Could you check a few things on this model? Use its own coordinates, in mm. Coordinates: 2 decimals unless noted, no trailing zeros. Loops run counter-clockwise (first coordinate to the right, second up) from the corner with the lowest first, then second, coordinate; pieces in that order, holes last. Notation, with made-up numbers: (-23, -13.5) - (-5, -13.5) arc R5 ccw to (-5, -7.5) - close; hole circle Ø2 at (58.5, 44). An arc over 180 degrees is marked (long way). Put each result on its own line as item: value. Start each with the question number.
```python
from build123d import *

# Parameters (mm, degrees)
SKETCH_1_R      = 5
SKETCH_1_R_2    = 2
EXTRUDE_1_DEPTH = 5


with BuildPart() as part:
    # 草图1 → 凸台-拉伸1 (new body)
    with BuildSketch(Plane(origin=(0, 0, 0), x_dir=(0, 0, -1), z_dir=(1, 0, 0))):
        with BuildLine():
            Line((-7, 33), (-7, 0))
            Line((-7, 0), (7, 0))
            Line((7, 0), (7, 33))
            ThreePointArc((7, 33), (0, 40), (-7, 33))
        make_face()
        with Locations((0, 33)):
            Circle(SKETCH_1_R, mode=Mode.SUBTRACT)
        with Locations((0, 13)):
            Circle(SKETCH_1_R_2, mode=Mode.SUBTRACT)
        with Locations((0, 7)):
            Circle(SKETCH_1_R_2, mode=Mode.SUBTRACT)
    extrude(amount=EXTRUDE_1_DEPTH)


solid = part.part
```
(1) I need wall thicknesses on L1, parallel to Y at x = 3.6, z = 0; L2, parallel to Y at x = 3.8, z = -1.5; L3, parallel to Z at x = 0.9, y = 31. Which ranges of each line are inside material? Lowest first, please. Write a range as [from, to].
(2) For pin 1 Ø2 at (x, z) = (2, -4.5) entering from +Y; pin 2 Ø1.5 at (x, z) = (1, 4) entering from +Y; pin 3 Ø1.5 at (x, z) = (2, -1) entering from -Y, each with a flat end and sliding along its axis, tell me the tip position at first contact or that it passes through.
(3) I want a section at A-A on y = 7. List the corners of the cut face in (x, z) for me.
(4) I want a section at B-B on z = 0. List the corners of the cut face in (x, y) for me, and give its area (3 significant figures).
(5) I want a section at C-C on x = 3.25. List the corners of the cut face in (y, z) for me, and give its area (3 significant figures).
(6) I want a section at D-D on z = -1.5. List the corners of the cut face in (x, y) for me, and give its area (3 significant figures).
(7) If we mould it in two halves opening along Y, with no side actions, what happens to faces 1 (the cylindrical face through (2, 40, 0)), 2 (the cylindrical face through (2, 37, -3)), 3 (the cylindrical face through (2, 15, 0)), 4 (the flat face through (2, 0, 0))? For each: pulls with the +Y half, pulls with the -Y half, needs draft (parallel to the pull), parting line crosses it, or undercut.
Answer sheet:
1. L1: y = [0, 5], [9, 11], [15, 28], [38, 40]
1. L2: y = [0, 5.68], [8.32, 11.68], [14.32, 28.23], [37.77, 39.84]
1. L3: z = [-7, -4.58], [4.58, 7]
2. pin 1: stops at y = 39.06
2. pin 2: stops at y = 39.2
2. pin 3: stops at y = 0
3. outline: (0, -7) - (5, -7) - (5, -2) - (0, -2) - close; (0, 2) - (5, 2) - (5, 7) - (0, 7) - close
4. outline: (0, 0) - (5, 0) - (5, 5) - (0, 5) - close; (0, 9) - (5, 9) - (5, 11) - (0, 11) - close; (0, 15) - (5, 15) - (5, 28) - (0, 28) - close; (0, 38) - (5, 38) - (5, 40) - (0, 40) - close
4. area: 110 mm^2
5. outline: (0, -7) - (33, -7) arc R7 ccw to (33, 7) - (0, 7) - close; hole circle Ø4 at (7, 0); hole circle Ø4 at (13, 0); hole circle Ø10 at (33, 0)
5. area: 435 mm^2
6. outline: (0, 0) - (5, 0) - (5, 5.68) - (0, 5.68) - close; (0, 8.32) - (5, 8.32) - (5, 11.68) - (0, 11.68) - close; (0, 14.32) - (5, 14.32) - (5, 28.23) - (0, 28.23) - close; (0, 37.77) - (5, 37.77) - (5, 39.84) - (0, 39.84) - close
6. area: 125 mm^2
7. face 1: pulls with the +Y half
7. face 2: undercut
7. face 3: undercut
7. face 4: pulls with the -Y half
